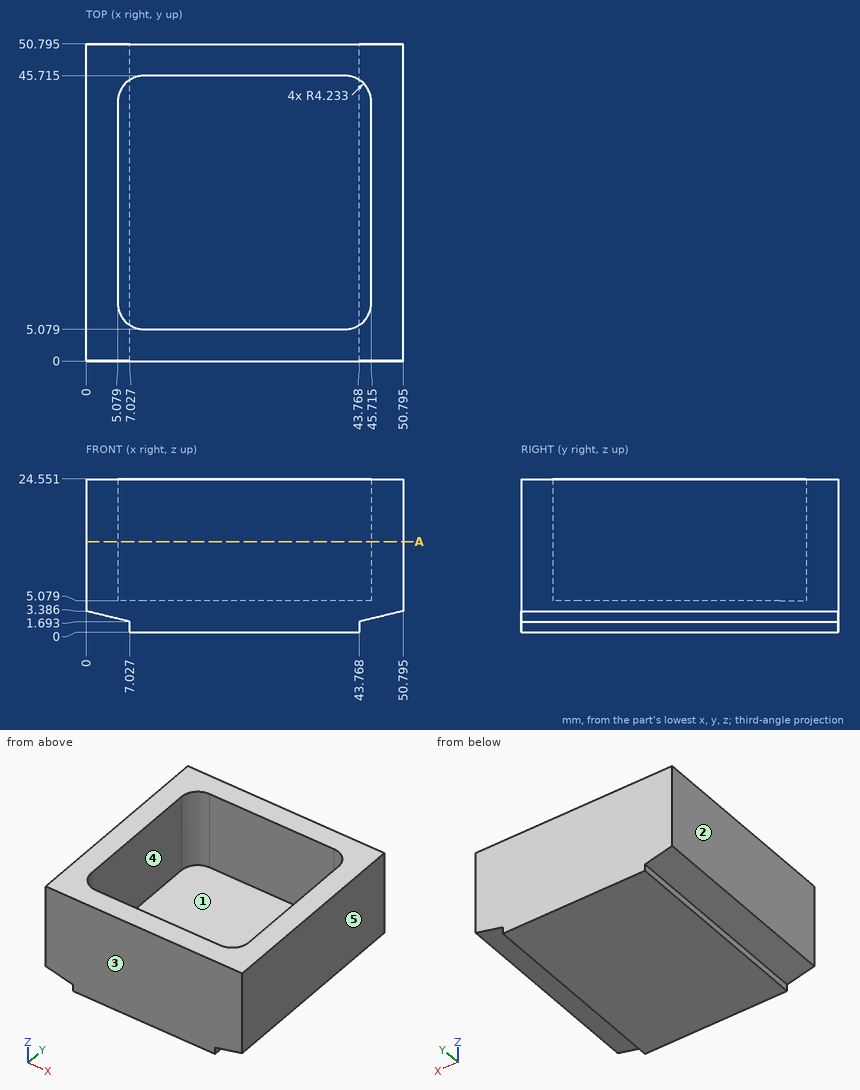
Design review of the part shown in the three views and the two pictorial views. Dimensions are in mm from the part's minimum x, y and z. A direction names the side the tool comes from. Round coordinates to 2 decimals unless told otherwise and drop trailing zeros. Loops run counter-clockwise (first coordinate to the right, second up) from the corner with the lowest first, then second, coordinate; pieces in that order, holes last.
Q1. Machinability: for the marked faces 1 and 2, which of the approach directions +Z, -Z, +X, -X, +Y, -Y give a long, thin tool a straight path to every point of the face, cutting with its end or side? Answer none if there is none.
Result sheet:
face 1: +Z
face 2: +Z, -Z, -X, +Y, -Y
Q2. Add section A-A on z = 14.5. Write out the cut boundary in (x, y) (1 decimal).
Result sheet:
outline: (0, 0) - (50.8, 0) - (50.8, 50.8) - (0, 50.8) - close; hole (5.1, 9.3) arc R4.2 ccw to (9.3, 5.1) - (41.5, 5.1) arc R4.2 ccw to (45.7, 9.3) - (45.7, 41.5) arc R4.2 ccw to (41.5, 45.7) - (9.3, 45.7) arc R4.2 ccw to (5.1, 41.5) - close
Q3. Mouldability with a two-part tool opening along Y and no side actions: class the marked faces 3, 4 and 5 as +Y half, -Y half, draft (parallel to the pull), parting line (faces both ways), or undercut.
Result sheet:
face 3: -Y half
face 4: undercut
face 5: draft
Q4. Insertion check: pin 1 Ø2 at (x, y) = (29.5, 15) entering from +Z; pin 2 Ø1.4 at (y, z) = (30.5, 0.5) entering from -X; pin 3 Ø0.5 at (y, z) = (24, 0.5) entering from +X. Each pin has a flat end and moves straight along its axis. Give the tip position at first contact, or say it passes through.
Result sheet:
pin 1: stops at z = 5.08
pin 2: stops at x = 7.03
pin 3: stops at x = 43.77
Q5. To check wall thickness, follow line 1 along X through (y, z) = (20, 15.25) (1 decimal); line 2 along Z through (x, y) = (20.5, 8). State the ranges of each line that lie inside material, in increasing order.
Result sheet:
line 1: x = 0 to 5.1, 45.7 to 50.8
line 2: z = 0 to 5.08
